Build history of the part. All positions in model axes, mm. Round coordinates to 2 decimals unless told otherwise and drop trailing zeros. Loops run counter-clockwise (first coordinate to the right, second up) from the corner with the lowest first, then second, coordinate; pieces in that order, holes last. Notation, with made-up numbers: (33.5, 32.5) - (79.5, 32.5) arc R33 cw to (79.5, 69.5) - close; hole circle Ø6 at (-36.5, 9.5). An arc over 180 degrees is marked (long way). Use a Markdown table: item, result.
from build123d import *

# Parameters (mm, degrees)
EXTRUDE_1_DEPTH     = 5
SKETCH_2_R          = 3.25
CUT_EXTRUDE_1_DEPTH = 19
SKETCH_3_R          = 1.4
SKETCH_3_R_2        = 5
CUT_EXTRUDE_3_DEPTH = 16.3


with BuildPart() as part:
    # 草图1 → 凸台-拉伸1 (new body)
    with BuildSketch(Plane(origin=(0, 0, 0), x_dir=(1, 0, 0), z_dir=(0, 1, 0))):
        with BuildLine():
            Line((-17.564991461, 54.578581424), (67.059916818, 223.42374787))
            ThreePointArc((67.059916818, 223.42374787), (114.908570146, 233.021342221), (136.424164559, 189.21852679))
            Line((136.424164559, 189.21852679), (53.992344711, 19.291894357))
            ThreePointArc((53.992344711, 19.291894357), (50.907753569, 10.392547603), (49.989622613, 1.018641763))
            ThreePointArc((49.989622613, 1.018641763), (-22.113685441, -44.844006469), (-29.624956892, 40.278554209))
            ThreePointArc((-29.624956892, 40.278554209), (-22.747275075, 46.713658557), (-17.564991461, 54.578581424))
        make_face()
    extrude(amount=EXTRUDE_1_DEPTH)

    # 草图2 → 切除-拉伸1 (cut)
    with BuildSketch(Plane.XZ):
        with Locations(Location((12.651398898, 37.946569093, 0), (0, 0, 270))):
            Circle(SKETCH_2_R)
        with Locations((81.596428252, -36.190269417)):
            Circle(SKETCH_2_R)
        with Locations((7.459589742, -105.135298771)):
            Circle(SKETCH_2_R)
        with Locations((-61.485439612, -30.998460261)):
            Circle(SKETCH_2_R)
    extrude(amount=-CUT_EXTRUDE_1_DEPTH, mode=Mode.SUBTRACT)

    # 草图3 → 切除-拉伸3 (cut)
    with BuildSketch(Plane.XZ):
        with Locations(Location((-16.224862373, 32.454617251, 0), (0, 0, 270))):
            Circle(SKETCH_3_R)
        with Locations(Location((-19.803218354, 21.72170672, 0), (0, 0, 270))):
            Circle(SKETCH_3_R)
        with Locations(Location((-12.647585098, 25.298983995, 0), (0, 0, 270))):
            Circle(SKETCH_3_R_2)
        with Locations(Location((-5.491951842, 28.876261271, 0), (0, 0, 270))):
            Circle(SKETCH_3_R)
        with Locations(Location((-9.070307822, 18.143350739, 0), (0, 0, 270))):
            Circle(SKETCH_3_R)
    extrude(amount=-CUT_EXTRUDE_3_DEPTH, mode=Mode.SUBTRACT)


solid = part.part
Q1. Pull direction X, two halves, no side cores. Call faces 1 (the face through (-22.833, 2.465, -46.613)), 2 (the face through (12.794, 2.465, 41.193)), 3 (the face through (95.785, 2.465, -105.445)): pulls with the +X half, pulls with the -X half, needs draft (parallel to the pull), parting line crosses it, or undercut.
Results found:
| item | result |
|---|---|
| face 1 | pulls with the -X half |
| face 2 | undercut |
| face 3 | pulls with the +X half |
Q2. Cut at B-B, the plane x = 0. List the corners of the cut face in (y, z).
Results found:
| item | result |
|---|---|
| outline | (0, -89.62) - (5, -89.62) - (5, 50) - (0, 50) - close |
Q3. Drop a flat-ended pin along its axis: pin 1 (1.5 mm diameter, centred on y = 3, z = -48.5, fed in from +X). Give the stop position or say it passes through.
Results found:
| item | result |
|---|---|
| pin 1 | stops at x = 68.53 |
Q4. Probe line 1 (Z direction, x = -16, y = 1.1); line 2 (X direction, y = 4.5, z = 38); line 3 (Z direction, x = 12.5, y = 2.7). List the from-to ranges inside material, lowest first.
Results found:
| item | result |
|---|---|
| line 1 | z = -57.7 to 21.59, 29.01 to 31.07, 33.84 to 47.37 |
| line 2 | x = -32.5 to 9.4, 15.9 to 32.5 |
| line 3 | z = -114.56 to 34.7, 41.19 to 48.41 |
Q5. Cut at A-A, the plane y = 2.6. List the corners of the cut face in (x, z) (3 decimals), plus the area to 3 significant figures.
Results found:
| item | result |
|---|---|
| outline | (-29.625, -40.279) arc R40 cw to (-17.565, -54.579) - (6.26, -102.115) arc R3.25 cw to (9.162, -107.904) - (67.06, -223.424) arc R40 ccw to (136.424, -189.219) - (53.992, -19.292) arc R40 cw to (49.99, -1.019) arc R50 ccw (long way) to start; hole circle Ø2.8 at (-19.803, 21.722); hole circle Ø10 at (-12.648, 25.299); hole circle Ø2.8 at (-16.225, 32.455); hole circle Ø2.8 at (-9.07, 18.143); hole circle Ø2.8 at (-5.492, 28.876); hole circle Ø6.5 at (12.651, 37.947) |
| area | 24,000 mm2 |
Q6. Cut at C-C, the plane z = -184.5. List the corners of the cut face in (x, y), plus the area to 3 significant figures.
Results found:
| item | result |
|---|---|
| outline | (47.55, 0) - (134.14, 0) - (134.14, 5) - (47.55, 5) - close |
| area | 433 mm2 |
